Geometry check sheet. Reference: the model listing, model coordinates, mm. Face numbers are marked on the shaded views. A direction names the side the tool comes from. Coordinates: 2 decimals unless noted, no trailing zeros. Order: outer loops, then holes, each group sorted by start corner. A loop starts at its lowest first (then second) coordinate and runs counter-clockwise, first axis right, second up. Notation, with made-up numbers: (-8.75, -27) -> (20.25, -27) arc R19 ccw to (20.25, -10) -> close; hole circle Ø10 at (8.5, 51.25). An arc over 180 degrees is marked (long way). Answer in a Markdown table with one row per item. Add a question column.
```python
from build123d import *

# Parameters (mm, degrees)
EXTRUDE_1_DEPTH     = 40
CUT_EXTRUDE_START   = -4
CUT_EXTRUDE_2_DEPTH = 50
CUT_EXTRUDE_3_DEPTH = 8


with BuildPart() as part:
    # 草图3 → 凸台-拉伸1 (new, symmetric)
    with BuildSketch(Plane.XY):
        Polygon((14, 42.647058824), (-14, 42.647058824), (-25, -7.352941176), (25, -7.352941176), align=None)
    extrude(amount=EXTRUDE_1_DEPTH, both=True)

    # 草图4 → 切除-拉伸2 (cut)
    with BuildSketch(Plane(origin=(0, 0, 0), x_dir=(0, 0, -1), z_dir=(1, 0, 0)).offset(CUT_EXTRUDE_START)):
        Polygon((13, 42.647058824), (-13, 42.647058824), (-27.558809371, 2.647058824), (27.558809371, 2.647058824), align=None)
    cut_extrude_2 = extrude(amount=-CUT_EXTRUDE_2_DEPTH, mode=Mode.SUBTRACT)

    # 镜向1: 切除-拉伸2 across plane
    add(cut_extrude_2.mirror(Plane(origin=(0, 0, 0), x_dir=(0, 0, 1), z_dir=(1, 0, 0))), mode=Mode.SUBTRACT)

    # 草图6 → 切除-拉伸3 (cut)
    with BuildSketch(Plane.ZY.offset(4)):
        with BuildLine():
            Line((-12, 36.647058824), (12, 36.647058824))
            ThreePointArc((12, 36.647058824), (0, 24.647058824), (-12, 36.647058824))
        make_face()
    extrude(amount=-CUT_EXTRUDE_3_DEPTH, mode=Mode.SUBTRACT)


solid = part.part
```
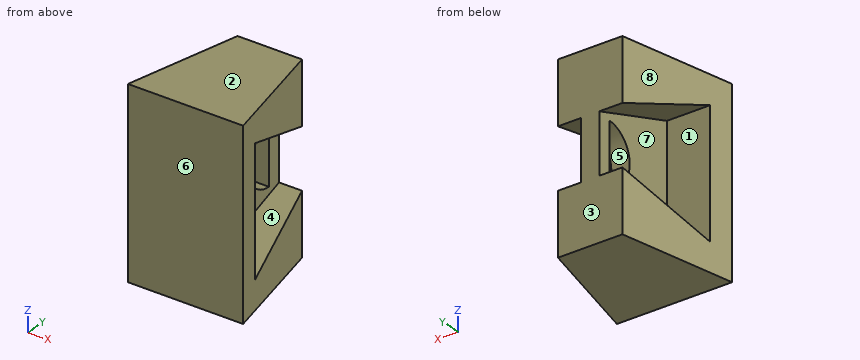
(1) Go/stop test with flat-tipped pins: P1, Ø20, axis at y = 32.5, z = 2, coming from the +X side; P2, Ø4, axis at y = 32.5, z = -16, coming from the +X side; P3, Ø8, axis at y = 29, z = -21.5, coming from the +X side. Record where each tip stops, or that it passes through.
(2) Cross-section at B-B (x = -8). Enter the section's corners in (y, z).
(3) Cross-section at A-A (z = 0). Enter the section's corners in (x, y), plus the area to 3 significant figures.
(4) Mould release check, pull along Y, two halves, no side actions. Record for the marked faces 1, 2 and 3: +Y half, -Y half, draft (parallel to the pull), parting line (faces both ways), or undercut.
(5) Cross-section at C-C (y = 31.5). Enter the section's corners in (x, z), plus the area to 3 significant figures.
(6) Cross-section at D-D (y = 38). Enter the section's corners in (x, z), plus the area to 3 significant figures.
(7) Access from +Z, -Z, +X, -X, +Y, -Y to the whole of each face (thin tool, end or side, straight path). Record for the marked faces 4, 5, 6, 7 and 8.
(8) Scan lines: line 1 along X through (y, z) = (7, -13); line 2 along Y through (x, z) = (17, 17); line 3 along Z through (x, y) = (-19, 15.5). Record each from-to range of solid material in increasing order.
Checks:
| question | item | result |
|---|---|---|
| 1 | P1 | x = 4 |
| 1 | P2 | x = 16.57 |
| 1 | P3 | x = 17.88 |
| 2 | outline | (-7.35, -40) -> (42.65, -40) -> (42.65, -13) -> (2.65, -27.56) -> (2.65, 27.56) -> (42.65, 13) -> (42.65, 40) -> (-7.35, 40) -> close |
| 3 | outline | (-25, -7.35) -> (25, -7.35) -> (22.8, 2.65) -> (4, 2.65) -> (4, 24.65) -> (-4, 24.65) -> (-4, 2.65) -> (-22.8, 2.65) -> close; (-4, 36.65) -> (4, 36.65) -> (4, 42.65) -> (-4, 42.65) -> close |
| 3 | area | 702 mm² |
| 4 | face 1 | undercut |
| 4 | face 2 | draft |
| 4 | face 3 | +Y half |
| 5 | outline | (-16.45, -40) -> (16.45, -40) -> (16.45, -17.06) -> (4, -17.06) -> (4, -10.84) -> (-4, -10.84) -> (-4, -17.06) -> (-16.45, -17.06) -> close; (-16.45, 17.06) -> (-4, 17.06) -> (-4, 10.84) -> (4, 10.84) -> (4, 17.06) -> (16.45, 17.06) -> (16.45, 40) -> (-16.45, 40) -> close |
| 5 | area | 1,610 mm² |
| 6 | outline | (-15.02, -40) -> (15.02, -40) -> (15.02, -14.69) -> (4, -14.69) -> (4, 14.69) -> (15.02, 14.69) -> (15.02, 40) -> (-15.02, 40) -> (-15.02, 14.69) -> (-4, 14.69) -> (-4, -14.69) -> (-15.02, -14.69) -> close |
| 6 | area | 1,760 mm² |
| 7 | face 4 | +X |
| 7 | face 5 | +X, -X |
| 7 | face 6 | +Z, -Z, +X, -X, -Y |
| 7 | face 7 | -X |
| 7 | face 8 | +Z, -Z, -X, +Y |
| 8 | line 1 | -4 to 4 |
| 8 | line 2 | -7.35 to 2.65 |
| 8 | line 3 | -40 to -22.88, 22.88 to 40 |
